Part model, mm, in its own coordinate system. A direction names the side the tool comes from. Round coordinates to 2 decimals unless told otherwise and drop trailing zeros. Loops run counter-clockwise (first coordinate to the right, second up) from the corner with the lowest first, then second, coordinate; pieces in that order, holes last. Notation, with made-up numbers: (42, -21.5) -> (48, -21.5) arc R17 cw to (48, 8.5) -> close; hole circle Ø9 at (80, 45.25). An arc over 180 degrees is marked (long way). Answer as a JSON object with one key per item and string values. Group by question number.
Autodesk Inventor part; units mm, degrees
ref_plane "YZ Plane" through (0, 0, 0) normal (1, 0, 0) x (0, 1, 0)
ref_plane "XZ Plane" through (0, 0, 0) normal (0, 1, 0) x (-1, 0, 0)
ref_plane "XY Plane" through (0, 0, 0) normal (0, 0, 1) x (1, 0, 0)
sketch "Sketch1" plane through (0, 0, 0) normal (0, 1, 0) x (-1, 0, 0)
  circle A0 centre (0, 0) radius 29
  line L0 (-8.1695, -14.15) -> (-16.339, 0)
  line L1 (-16.339, 0) -> (-8.1695, 14.15)
  line L2 (-8.1695, 14.15) -> (8.1695, 14.15)
  line L3 (8.1695, 14.15) -> (16.339, 0)
  line L4 (16.339, 0) -> (8.1695, -14.15)
  line L5 (8.1695, -14.15) -> (-8.1695, -14.15)
  dimension "d0" = 58
  dimension "d1" = 28.3
extrude "Plate1" add sketch "Sketch1" along normal blind 1
sketch "Sketch2" plane through (0, 0, 0) normal (0, 1, 0) x (-1, 0, 0)
  point P0 (0, 0)
  point P1 (22, 0)
  point P2 (-22, 0)
  dimension "d3" = 22
  dimension "d4" = 22
hole "Hole1" at (-22, 0, 0) at (22, 0, 0) direction (0, 1, 0) diameter 3.3 end through all
sketch "Sketch3" plane through (0, 1, 0) normal (0, 1, 0) x (1, 0, 0)
  line L0 (0, 0) -> (8.5176, 0)
  line L1 (0, 0) -> (0, 7.5276)
  line L2 (-8.75, 24) -> (8.75, 24)
  line L3 (8.75, 24) -> (8.75, 22.5)
  line L4 (8.75, 22.5) -> (-8.75, 22.5)
  line L5 (-8.75, 22.5) -> (-8.75, 24)
  line L6 (0.75, 42.5) -> (-0.75, 42.5)
  line L7 (-0.75, 42.5) -> (-0.75, 22.5)
  line L8 (-0.75, 22.5) -> (0.75, 22.5)
  line L9 (0.75, 22.5) -> (0.75, 42.5)
  line L10 (-8.75, -24) -> (8.75, -24)
  line L11 (8.75, -24) -> (8.75, -22.5)
  line L12 (8.75, -22.5) -> (-8.75, -22.5)
  line L13 (-8.75, -22.5) -> (-8.75, -24)
  line L14 (0.75, -42.5) -> (-0.75, -42.5)
  line L15 (-0.75, -42.5) -> (-0.75, -22.5)
  line L16 (-0.75, -22.5) -> (0.75, -22.5)
  line L17 (0.75, -22.5) -> (0.75, -42.5)
  line L18 (-27, 7.5) -> (-18.5, 7.5)
  line L19 (-18.5, 7.5) -> (-18.5, 6)
  line L20 (-18.5, 6) -> (-27, 6)
  line L21 (-27, 6) -> (-27, 7.5)
  line L22 (-18.5, 6) -> (-20, 6)
  line L23 (-20, 6) -> (-20, 20)
  line L24 (-20, 20) -> (-18.5, 20)
  line L25 (-18.5, 20) -> (-18.5, 6)
  line L26 (27, 7.5) -> (18.5, 7.5)
  line L27 (18.5, 7.5) -> (18.5, 6)
  line L28 (18.5, 6) -> (27, 6)
  line L29 (27, 6) -> (27, 7.5)
  line L30 (18.5, 6) -> (20, 6)
  line L31 (20, 6) -> (20, 20)
  line L32 (20, 20) -> (18.5, 20)
  line L33 (18.5, 20) -> (18.5, 6)
  line L34 (-27, -7.5) -> (-18.5, -7.5)
  line L35 (-18.5, -7.5) -> (-18.5, -6)
  line L36 (-18.5, -6) -> (-27, -6)
  line L37 (-27, -6) -> (-27, -7.5)
  line L38 (-18.5, -6) -> (-20, -6)
  line L39 (-20, -6) -> (-20, -20)
  line L40 (-20, -20) -> (-18.5, -20)
  line L41 (-18.5, -20) -> (-18.5, -6)
  line L42 (18.5, -20) -> (18.5, -6)
  line L43 (20, -6) -> (20, -20)
  line L44 (20, -20) -> (18.5, -20)
  line L45 (18.5, -7.5) -> (18.5, -6)
  line L46 (18.5, -6) -> (20, -6)
  line L47 (27, -6) -> (27, -7.5)
  line L48 (27, -7.5) -> (18.5, -7.5)
  line L49 (18.5, -6) -> (27, -6)
  point P0 (0, 22.5)
  point P1 (0, -22.5)
  dimension "d12" = 1.5
  dimension "d13" = 1.5
  dimension "d14" = 22.5
  dimension "d15" = 17.5
  dimension "d16" = 20
  dimension "d17" = 1.5
  dimension "d18" = 1.5
  dimension "d19" = 8.5
  dimension "d20" = 14
  dimension "d21" = 6
  dimension "d22" = 18.5
extrude "Cut1" cut sketch "Sketch3" against normal blind 1
equation "\"d10\" = Thickness"
equation "\"d23\" = Thickness"
equation "\"BendRadius\" = Thickness"
equation "\"BendReliefWidth\" = Thickness"
equation "\"BendReliefDepth\" = 0.5 * Thickness"
equation "\"CornerReliefSize\" = 4 * Thickness"
equation "\"MinimumRemnant\" = 2 * Thickness"
equation "\"TransitionRadius\" = BendRadius"
equation "\"JacobiRadiusSize\" = BendRadius"
equation "\"GapSize\" = Thickness"
equation "\"d2\" = BendRadius"
properties part number "Luxcan centrador lente 38"
Item 1: Band-saw the part on B-B, the plane z = 15. List the corners of the cut face in (x, y), plus the area to 3 significant figures.
Item 2: Band-saw the part on C-C, the plane x = -22. List the corners of the cut face in (y, z).
Item 3: Which spindle directions (+Z, -Z, +X, -X, +Y, -Y) get a long thin tool onto all of the face, cutting with end or side? Do faces 4 (the face through (12.31, 0.49, 6.98)), 5 (the face through (13.3, 1, -6)). Say none if no direction does.
Item 4: Drill centre lines: line 1 (X direction, y = 0.6, z = 0); line 2 (Z direction, x = -22, y = 0.75); line 3 (Z direction, x = 5, y = 0.8). Where is each one in solid material? Low to high.
Item 5: Band-saw the part on A-A, the plane x = 0. List the corners of the cut face in (y, z), plus the area to 3 significant figures.
Item 6: Two-plate mould, pull along Z, no slides. Class faces 1 (the face through (13.3, 0, -6)), 2 (the face through (-28.993, 0.493, 0.627)), 3 (the face through (20.364, 0.507, 0.215)): pulls with the +Z half, pulls with the -Z half, needs draft (parallel to the pull), parting line crosses it, or undercut.
Item 7: Drop flat-ended pins along their axis: pin 1 Ø0.5 at (x, y) = (22.5, 0.5) entering from -Z; pin 2 Ø0.5 at (x, y) = (4, 0.5) entering from -Z; pin 3 Ø0.5 at (x, y) = (19, 0.5) entering from +Z. Give the stop position or say it passes through.
Item 8: Band-saw the part on D-D, the plane z = 4. List the corners of the cut face in (x, y).
Entries:
{
 "1": {"outline": "(-24.82, 0) -> (-20, 0) -> (-20, 1) -> (-24.82, 1) -> close; (-18.5, 0) -> (18.5, 0) -> (18.5, 1) -> (-18.5, 1) -> close; (20, 0) -> (24.82, 0) -> (24.82, 1) -> (20, 1) -> close", "area": "46.6 mm²"},
 "2": {"outline": "(0, -18.89) -> (1, -18.89) -> (1, -7.5) -> (0, -7.5) -> close; (0, -6) -> (1, -6) -> (1, -1.65) -> (0, -1.65) -> close; (0, 1.65) -> (1, 1.65) -> (1, 6) -> (0, 6) -> close; (0, 7.5) -> (1, 7.5) -> (1, 18.89) -> (0, 18.89) -> close"},
 "3": {"face 4": "+Y, -Y", "face 5": "+Z, -Z, +X, -X, +Y"},
 "4": {"line 1": "-29 to -23.65, -20.35 to -16.34, 16.34 to 20.35, 23.65 to 29", "line 2": "-18.89 to -7.5, -6 to -1.65, 1.65 to 6, 7.5 to 18.89", "line 3": "-28.57 to -24, -22.5 to -14.15, 14.15 to 22.5, 24 to 28.57"},
 "5": {"outline": "(0, -22.5) -> (1, -22.5) -> (1, -14.15) -> (0, -14.15) -> close; (0, 14.15) -> (1, 14.15) -> (1, 22.5) -> (0, 22.5) -> close", "area": "16.7 mm²"},
 "6": {"face 1": "needs draft", "face 2": "parting line crosses it", "face 3": "undercut"},
 "7": {"pin 1": "z = -18.6", "pin 2": "z = -28.76", "pin 3": "z = 22.12"},
 "8": {"outline": "(-28.72, 0) -> (-14.03, 0) -> (-14.03, 1) -> (-28.72, 1) -> close; (14.03, 0) -> (28.72, 0) -> (28.72, 1) -> (14.03, 1) -> close"}
}
